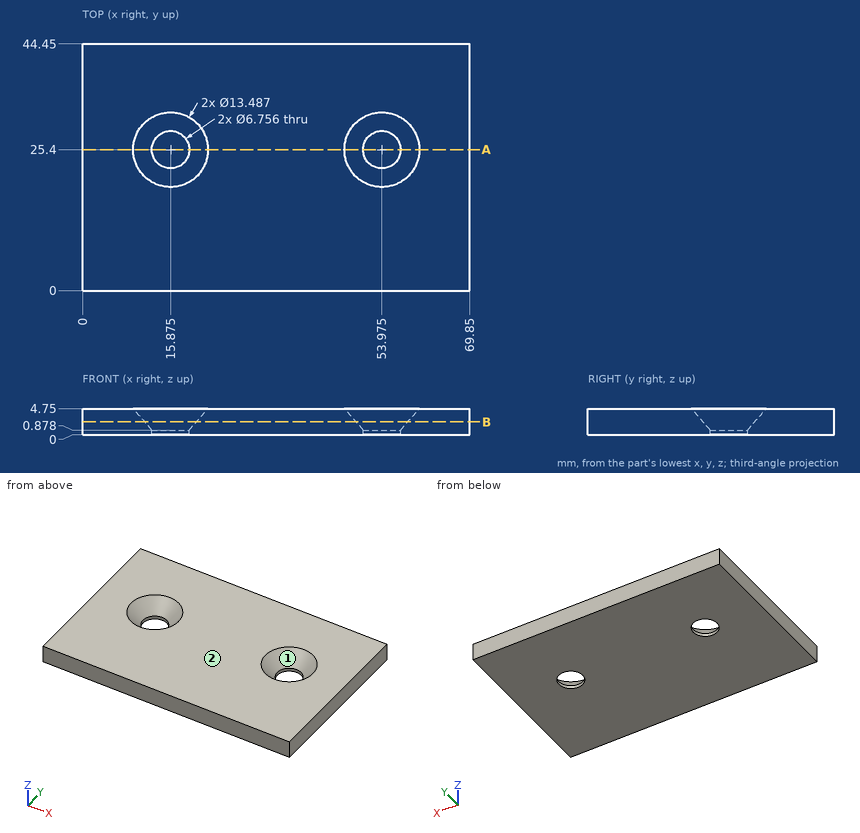
Study the drawing (mm; zero at the part's minimum x, y, z) and answer. Round coordinates to 2 decimals unless told otherwise and drop trailing zeros. Order: outer loops, then holes, each group sorted by start corner. A loop starts at its lowest first (then second) coordinate and runs counter-clockwise, first axis right, second up. Notation, with made-up numbers: M -21.5,0.25 L -3.5,0.25 A20 ccw -3.5,36.25 Z; hole C 73.5,-34 d9. An arc over 180 degrees is marked long. One line per item, written item: value.
Q1. Straight lines are drawn through the part: line 1 (X direction, y = 25.4, z = 0.5); line 2 (Y direction, x = 51, z = 0.85); line 3 (Y direction, x = 53, z = 4.55). For each, find the intervals that lie inside material, in ascending order.
Derived:
line 1: 0 to 12.5, 19.25 to 50.6, 57.35 to 69.85
line 2: 0 to 23.8, 27 to 44.45
line 3: 0 to 18.9, 31.9 to 44.45
Q2. Find section B-B on z = 2.35. Give the number of separate pieces and of enclosed holes in the cut face, then the cut area to 3 significant figures.
Derived:
separate pieces: 1
enclosed holes: 2
area: 2,970 mm²
Q3. A flat-ended cylindrical pin translates along its axis: pin 1 (9 mm diameter, centred on x = 15.875, y = 25.4, fed in from +Z). Find the tip coordinate at first contact, or state that the pin passes through.
Derived:
pin 1: z = 2.17
Q4. Determine the mould class of the marked faces 1 and 2 for opening direction X: released by +X, released by -X, zero draft, split by the parting line, or undercut.
Derived:
face 1: undercut
face 2: zero draft
Q5. Find section A-A on y = 25.4. Write down the section's boundary in (x, z).
Derived:
outline: M 0,0 L 12.5,0 L 12.5,0.88 L 9.13,4.75 L 0,4.75 Z; M 19.25,0 L 50.6,0 L 50.6,0.88 L 47.23,4.75 L 22.62,4.75 L 19.25,0.88 Z; M 57.35,0 L 69.85,0 L 69.85,4.75 L 60.72,4.75 L 57.35,0.88 Z
